Build history of the part. All positions in model axes, mm. Face numbers are marked on the shaded views. A direction names the side the tool comes from. Give positions to 0.01 mm unless a question says otherwise; leave off trailing zeros. Write each loop counter-clockwise with the first axis right and the second up, starting at its lowest first coordinate (ties: lowest second). Pieces come first, ordered by that corner, then holes.
from build123d import *

# Parameters (mm, degrees)
SKETCH1_W           = 22
SKETCH1_H           = 30
BOSS_EXTRUDE1_DEPTH = 8.7
SKETCH2_W           = 63.9
SKETCH2_H           = 41.5
SKETCH2_W_2         = 55.9
SKETCH2_H_2         = 33.5
BOSS_EXTRUDE2_DEPTH = 11.5
SKETCH3_R           = 5
SKETCH3_R_2         = 2
BOSS_EXTRUDE3_DEPTH = 8.5
SKETCH4_R           = 5
BOSS_EXTRUDE4_DEPTH = 3
FILLET2_R           = 15


with BuildPart() as part:
    # Sketch1 → Boss-Extrude1 (new body)
    with BuildSketch(Plane(origin=(0, 0, 0), x_dir=(1, 0, 0), z_dir=(0, 1, 0))):
        Polygon((-26.45, -16.75), (26.45, -16.75), (27.95, -16.75), (27.95, 16.75), (26.45, 16.75), (-26.45, 16.75), (-27.95, 16.75), (-27.95, -16.75), align=None)
        with Locations((-13.55, 0)):
            Rectangle(SKETCH1_W, SKETCH1_H, mode=Mode.SUBTRACT)
        with Locations((13.55, 0)):
            Rectangle(SKETCH1_W, SKETCH1_H, mode=Mode.SUBTRACT)
    extrude(amount=BOSS_EXTRUDE1_DEPTH)

    # Sketch2 → Boss-Extrude2 (add)
    with BuildSketch(Plane.XZ):
        Rectangle(SKETCH2_W, SKETCH2_H)
        Rectangle(SKETCH2_W_2, SKETCH2_H_2, mode=Mode.SUBTRACT)
    extrude(amount=-BOSS_EXTRUDE2_DEPTH)

    # Sketch3 → Boss-Extrude3 (add)
    # profile 1 of 5: a face of its own
    with BuildSketch(Plane(origin=(0, 11.5, 0), x_dir=(1, 0, 0), z_dir=(0, 1, 0))):
        with Locations((-32.95, 22.482050808)):
            Circle(SKETCH3_R)
        with Locations(Location((-32.95, 22.482050808, 0), (0, 0, 270))):
            Circle(SKETCH3_R_2, mode=Mode.SUBTRACT)
    # profile 2 of 5: a face of its own
    with BuildSketch(Plane(origin=(0, 11.5, 0), x_dir=(1, 0, 0), z_dir=(0, 1, 0))):
        with Locations((-32.95, -22.482050808)):
            Circle(SKETCH3_R)
        with Locations(Location((-32.95, -22.482050808, 0), (0, 0, 270))):
            Circle(SKETCH3_R_2, mode=Mode.SUBTRACT)
    # profile 3 of 5: a face of its own
    with BuildSketch(Plane(origin=(0, 11.5, 0), x_dir=(1, 0, 0), z_dir=(0, 1, 0))):
        with Locations((32.95, -22.482050808)):
            Circle(SKETCH3_R)
        with Locations(Location((32.95, -22.482050808, 0), (0, 0, 270))):
            Circle(SKETCH3_R_2, mode=Mode.SUBTRACT)
    # profile 4 of 5: a face of its own
    with BuildSketch(Plane(origin=(0, 11.5, 0), x_dir=(1, 0, 0), z_dir=(0, 1, 0))):
        with Locations((32.95, 22.482050808)):
            Circle(SKETCH3_R)
        with Locations(Location((32.95, 22.482050808, 0), (0, 0, 270))):
            Circle(SKETCH3_R_2, mode=Mode.SUBTRACT)
    # profile 5 of 5: a face of its own
    with BuildSketch(Plane(origin=(0, 11.5, 0), x_dir=(1, 0, 0), z_dir=(0, 1, 0))):
        with Locations((0, -22.75)):
            Circle(SKETCH3_R)
        with Locations(Location((0, -22.75, 0), (0, 0, 270))):
            Circle(SKETCH3_R_2, mode=Mode.SUBTRACT)
    extrude(amount=-BOSS_EXTRUDE3_DEPTH)

    # Sketch4 → Boss-Extrude4 (add)
    with BuildSketch(Plane.XZ.offset(-3)):
        with Locations((-32.95, -22.482050808)):
            Circle(SKETCH4_R)
        with Locations((-32.95, 22.482050808)):
            Circle(SKETCH4_R)
        with Locations((0, 22.75)):
            Circle(SKETCH4_R)
        with Locations((32.95, 22.482050808)):
            Circle(SKETCH4_R)
        with Locations((32.95, -22.482050808)):
            Circle(SKETCH4_R)
    extrude(amount=BOSS_EXTRUDE4_DEPTH)

    # Fillet2
    fillet2_edges = [part.edges().sort_by_distance(p)[0] for p in [
        (28.25958424, 5.75, 20.75),
        (31.95, 5.75, 17.583071322),
        (31.95, 5.75, -17.583071322),
        (28.25958424, 5.75, -20.75),
        (4.582575695, 5.75, 20.75),
        (-4.582575695, 5.75, 20.75),
        (-28.25958424, 5.75, -20.75),
        (-31.95, 5.75, -17.583071322),
        (-28.25958424, 5.75, 20.75),
        (-31.95, 5.75, 17.583071322),
    ]]
    fillet(fillet2_edges, radius=FILLET2_R)


solid = part.part
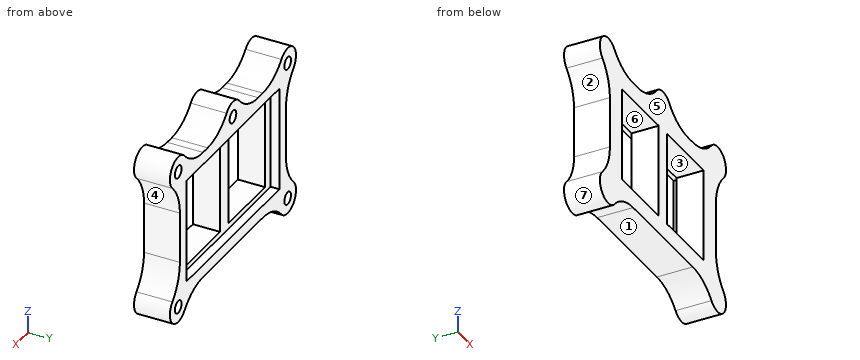
(1) Saw through at C-C, the plane x = -9. List the corners of the cut face in (y, z), plus the area to 3 significant figures.
(2) Saw through at D-D, the plane y = 2. List the corners of the cut face in (x, z), plus the area to 3 significant figures.
(3) Saw through at A-A, the plane z = 7. List the corners of the cut face in (x, y).
(4) Probe line 1 (Z direction, x = 14.5, y = 5); line 2 (X direction, y = 6.75, z = -1.5); line 3 (X direction, y = 1, z = 23). List the from-to ranges inside material, lowest first.
(5) Mould opens along X. For the marked faces 4, 5, 6 and 7 say: +X half, -X half, draft (parallel to the pull), parting line (faces both ways), or undercut.
(6) Saw through at B-B, the plane y = 6.75. Give the number of separate pieces and of enclosed holes in the cut face, plus the area to 3 significant figures.
(7) 3-axis set-ups, long thin cutter, end or side, ignore diameter. For the marked faces 1, 2 and 3: which of +Z, -Z, +X, -X, +Y, -Y reach the whole face in a straight line?
(8) Drop flat-ended pins along their axis: pin 1 (3.5 mm diameter, centred on x = 0, z = 22.75, fed in from -Y); pin 2 (5 mm diameter, centred on x = 10, y = 4.5, fed in from +Z); pin 3 (1.2 mm diameter, centred on x = 33.5, z = -23, fed in from +Y); pin 4 (4.5 mm diameter, centred on y = 6.5, z = -1, fed in from +X). Give the stop position or say it passes through.
Computed values:
1. outline: (0, -20.75) - (11.5, -20.75) - (11.5, -16.75) - (8.7, -16.75) - (8.7, -15) - (0, -15) - close; (0, 15) - (8.7, 15) - (8.7, 16.75) - (11.5, 16.75) - (11.5, 22.09) - (0, 22.09) - close
1. area: 138 mm2
2. outline: (-36.45, -18.91) arc R5 ccw (long way) to (-29.21, -25.8) arc R15 cw to (-17.98, -20.75) - (17.98, -20.75) arc R15 cw to (29.21, -25.8) arc R5 ccw (long way) to (36.45, -18.91) arc R15 cw to (31.95, -8.2) - (31.95, 8.2) arc R15 cw to (36.45, 18.91) arc R5 ccw (long way) to (29.21, 25.8) arc R15 cw to (17.98, 20.75) - (15.2, 20.75) arc R15 cw to (3.8, 26) arc R5 ccw to (-3.8, 26) arc R15 cw to (-15.2, 20.75) - (-17.98, 20.75) arc R15 cw to (-29.21, 25.8) arc R5 ccw (long way) to (-36.45, 18.91) arc R15 cw to (-31.95, 8.2) - (-31.95, -8.2) arc R15 cw to start; hole (-24.55, -15) - (-2.55, -15) - (-2.55, 15) - (-24.55, 15) - close; hole (2.55, -15) - (24.55, -15) - (24.55, 15) - (2.55, 15) - close
2. area: 1,790 mm2
3. outline: (-31.95, 0) - (-24.55, 0) - (-24.55, 8.7) - (-27.95, 8.7) - (-27.95, 11.5) - (-31.95, 11.5) - close; (-2.55, 0) - (2.55, 0) - (2.55, 8.7) - (-2.55, 8.7) - close; (24.55, 0) - (31.95, 0) - (31.95, 11.5) - (27.95, 11.5) - (27.95, 8.7) - (24.55, 8.7) - close
4. line 1: z = -20.75 to -15, 15 to 20.77
4. line 2: x = -31.95 to -24.55, -2.55 to 2.55, 24.55 to 31.95
4. line 3: x = -37.92 to -25.89, -7.3 to 7.3, 25.89 to 37.92
5. face 4: +X half
5. face 5: draft
5. face 6: undercut
5. face 7: undercut
6. separate pieces: 1
6. enclosed holes: 7
6. area: 1,730 mm2
7. face 1: -Z, +Y, -Y
7. face 2: -X, +Y, -Y
7. face 3: +Y, -Y
8. pin 1: stops at y = 0
8. pin 2: stops at z = 22.88
8. pin 3: stops at y = 3
8. pin 4: stops at x = 31.95
